Check sheet for the modelled part. Datum: model origin and axes. Units: mm. Face numbers are marked on the shaded views. A direction names the side the tool comes from. Round coordinates to 2 decimals unless told otherwise and drop trailing zeros. Write each loop counter-clockwise with the first axis right and the second up, starting at its lowest first coordinate (ties: lowest second). Pieces come first, ordered by that corner, then holes. Notation, with made-up numbers: (57, 62) -> (93, 62) arc R17 ccw to (93, 90) -> close; hole circle Ø5 at (-30, 31). An arc over 180 degrees is marked (long way). One line per item, written item: value.
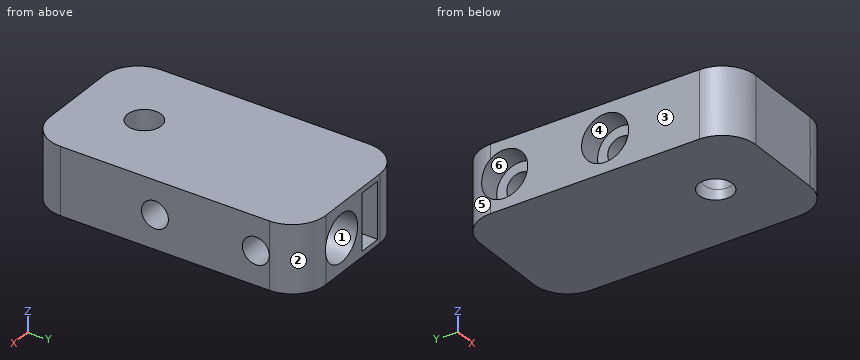
from build123d import *

# Parameters (mm, degrees)
CROQUIS1_W              = 10
CROQUIS1_H              = 41
SALIENTE_EXTRUIR1_DEPTH = 21.8
CROQUIS6_R              = 2
CORTAR_EXTRUIR2_DEPTH   = 21.8
CORTAR_EXTRUIR4_REACH   = 49.5
CROQUIS11_R             = 3.5
CROQUIS11_W             = 3.4
CROQUIS11_H             = 8.4
CORTAR_EXTRUIR5_REACH   = 49.5
CROQUIS12_R             = 2.5
REDONDEO1_R             = 5
CROQUIS13_R             = 3.5
CORTAR_EXTRUIR6_DEPTH   = 3.5
CROQUIS15_W             = 3.4
CROQUIS15_H             = 8.4
SALIENTE_EXTRUIR2_DEPTH = 13
CORTAR_EXTRUIR7_START   = -10
CROQUIS16_R             = 2.5
CORTAR_EXTRUIR7_DEPTH   = 10


with BuildPart() as part:
    # Croquis1 → Saliente-Extruir1 (new body)
    with BuildSketch(Plane(origin=(0, 0, 0), x_dir=(0, 0, -1), z_dir=(1, 0, 0))):
        with Locations((-5, -20.5)):
            Rectangle(CROQUIS1_W, CROQUIS1_H)
    extrude(amount=SALIENTE_EXTRUIR1_DEPTH)

    # Croquis6 → Cortar-Extruir2 (cut)
    with BuildSketch(Plane.ZY):
        with Locations((5, -22)):
            Circle(CROQUIS6_R)
        with Locations((5, -7)):
            Circle(CROQUIS6_R)
    extrude(amount=-CORTAR_EXTRUIR2_DEPTH, mode=Mode.SUBTRACT)

    # Croquis11 → Cortar-Extruir4 (cut, up to next)
    with BuildSketch(Plane.XZ.offset(41), mode=Mode.PRIVATE) as cortar_extruir4_sk1:
        with Locations(Location((13.4, 5, 0), (0, 0, 270))):
            Circle(CROQUIS11_R)
    cortar_extruir4_tool1 = extrude(cortar_extruir4_sk1.sketch, amount=-CORTAR_EXTRUIR4_REACH, mode=Mode.PRIVATE) & part.part
    # Croquis11 → Cortar-Extruir4 (cut, up to next)
    with BuildSketch(Plane.XZ.offset(41), mode=Mode.PRIVATE) as cortar_extruir4_sk2:
        with Locations((7.2, 5)):
            Rectangle(CROQUIS11_W, CROQUIS11_H)
    cortar_extruir4_tool2 = extrude(cortar_extruir4_sk2.sketch, amount=-CORTAR_EXTRUIR4_REACH, mode=Mode.PRIVATE) & part.part
    add(cortar_extruir4_tool1.solids().sort_by_distance((13.4, -41, 5))[0], mode=Mode.SUBTRACT)
    add(cortar_extruir4_tool2.solids().sort_by_distance((7.2, -41, 5))[0], mode=Mode.SUBTRACT)

    # Cortar-Extruir5: up to this face of the body (flat: up to its plane)
    cortar_extruir5_end = Plane(part.part.faces().sort_by_distance((10.9, -20.5, 10))[0])
    # Croquis12 → Cortar-Extruir5 (cut, up to the picked face)
    with BuildSketch(Plane(origin=(0, 0, 0), x_dir=(-1, 0, 0), z_dir=(0, 0, -1)), mode=Mode.PRIVATE) as cortar_extruir5_sk1:
        with Locations(Location((-10.9, -31, 0), (0, 0, 90))):
            Circle(CROQUIS12_R)
    cortar_extruir5_tool1 = split(extrude(cortar_extruir5_sk1.sketch, amount=-CORTAR_EXTRUIR5_REACH, mode=Mode.PRIVATE), bisect_by=cortar_extruir5_end, keep=Keep.BOTH, mode=Mode.PRIVATE)
    add(cortar_extruir5_tool1.solids().sort_by(Axis((10.9, -31, 0), (0, 0, 1)))[0], mode=Mode.SUBTRACT)

    # Redondeo1
    # the kernel refuses this fillet: 5 mm, written as the material it takes off along each edge
    with BuildSketch(Plane(origin=(21.8, -41, 22.5), x_dir=(0, 1, 0), z_dir=(0, 0, -1)), Plane(origin=(0, 0, -12.5), x_dir=(1, 0, 0), z_dir=(0, 0, 1))) as redondeo1_piece_1:
        with BuildLine():
            CenterArc((REDONDEO1_R, -REDONDEO1_R), REDONDEO1_R, 90, 90)
            Line((0, -REDONDEO1_R), (0, 0))
            Line((0, 0), (REDONDEO1_R, 0))
        make_face()
    extrude(amount=35, mode=Mode.SUBTRACT)
    with BuildSketch(Plane(origin=(21.8, 0, -12.5), x_dir=(-1, 0, 0), z_dir=(0, 0, 1)), Plane(origin=(0, -41, 22.5), x_dir=(0, 1, 0), z_dir=(0, 0, -1))) as redondeo1_piece_2:
        with BuildLine():
            CenterArc((REDONDEO1_R, REDONDEO1_R), REDONDEO1_R, 180, 90)
            Line((0, REDONDEO1_R), (0, 0))
            Line((0, 0), (REDONDEO1_R, 0))
        make_face()
    extrude(amount=35, mode=Mode.SUBTRACT)

    # Croquis13 → Cortar-Extruir6 (cut)
    with BuildSketch(Plane.ZY):
        with Locations((5, -7)):
            Circle(CROQUIS13_R)
        with Locations((5, -22)):
            Circle(CROQUIS13_R)
    extrude(amount=-CORTAR_EXTRUIR6_DEPTH, mode=Mode.SUBTRACT)

    # Croquis15 → Saliente-Extruir2 (add)
    with BuildSketch(Plane.XZ.offset(41)):
        with Locations((7.2, 5)):
            Rectangle(CROQUIS15_W, CROQUIS15_H)
        with BuildLine():
            ThreePointArc((16.8, 4.169337614), (16.9, 5), (16.8, 5.830662386))
            ThreePointArc((16.8, 5.830662386), (9.9, 5), (16.8, 4.169337614))
        make_face()
    extrude(amount=-SALIENTE_EXTRUIR2_DEPTH)

    # Croquis16 → Cortar-Extruir7 (cut)
    with BuildSketch(Plane.XY.offset(10).offset(CORTAR_EXTRUIR7_START)):
        with Locations(Location((10.9, -31, 0), (0, 0, 90))):
            Circle(CROQUIS16_R)
    extrude(amount=CORTAR_EXTRUIR7_DEPTH, mode=Mode.SUBTRACT)


solid = part.part
Item 1: Depth check by flat-ended pin: P1, Ø1, axis at x = 3, y = -24, coming from the -Z side; P2, Ø2, axis at y = -8, z = 5.5, coming from the -X side; P3, Ø1.7, axis at x = 7, z = 6, coming from the +Y side. Enter the tip coordinate at first touch or a pass-through.
Answer:
P1: stops at z = 0
P2: stops at x = 3.5
P3: stops at y = -28
Item 2: Tool access check on the marked faces 5 and 6. Record the directions out of +Z, -Z, +X, -X, +Y, -Y that give a thin tool (end or side, any length) a straight path to the whole face; none if there is none.
Answer:
face 5: +Z, -Z, -X, +Y
face 6: -X
Item 3: Sectioned sample at C-C on y = -13. Enter the section's corners in (x, z).
Answer:
outline: (0, 0) -> (21.8, 0) -> (21.8, 10) -> (0, 10) -> close; hole (5.5, 0.8) -> (8.9, 0.8) -> (8.9, 9.2) -> (5.5, 9.2) -> close; hole circle Ø7 at (13.4, 5)
Item 4: Sectioned sample at D-D on x = 17.5. Enter the section's corners in (y, z).
Answer:
outline: (-40.95, 0) -> (-0.05, 0) -> (-0.05, 10) -> (-40.95, 10) -> close; hole circle Ø4 at (-22, 5); hole circle Ø4 at (-7, 5)
Item 5: Sectioned sample at B-B on x = 9.5. Enter the section's corners in (y, z).
Answer:
outline: (-41, 0) -> (-33.07, 0) -> (-33.07, 10) -> (-41, 10) -> close; (-28.93, 0) -> (0, 0) -> (0, 10) -> (-28.93, 10) -> close; hole circle Ø4 at (-22, 5); hole circle Ø4 at (-7, 5)
Item 6: Mould release check, pull along X, two halves, no side actions. Record for the marked faces 1, 2, 3 and 4: pulls with the +X half, pulls with the -X half, needs draft (parallel to the pull), parting line crosses it, or undercut.
Answer:
face 1: undercut
face 2: pulls with the +X half
face 3: pulls with the -X half
face 4: needs draft
Item 7: Sectioned sample at A-A on y = -7. Enter the section's corners in (x, z), and give its area (3 significant figures).
Answer:
outline: (0, 0) -> (21.8, 0) -> (21.8, 3) -> (16.27, 3) arc R3.5 cw to (10.53, 3) -> (8.9, 3) -> (8.9, 0.8) -> (5.5, 0.8) -> (5.5, 3) -> (3.5, 3) -> (3.5, 1.5) -> (0, 1.5) -> close; (0, 8.5) -> (3.5, 8.5) -> (3.5, 7) -> (5.5, 7) -> (5.5, 9.2) -> (8.9, 9.2) -> (8.9, 7) -> (10.53, 7) arc R3.5 cw to (16.27, 7) -> (21.8, 7) -> (21.8, 10) -> (0, 10) -> close
area: 93.2 mm^2
Item 8: Thickness scan on line 1 (X direction, y = -16.5, z = 5); line 2 (X direction, y = -19.5, z = 5); line 3 (X direction, y = -31, z = 3.25). Record the ranges inside material, lowest first.
Answer:
line 1: x = 0 to 5.5, 8.9 to 9.9, 16.9 to 21.8
line 2: x = 3.5 to 5.5, 8.9 to 9.9, 16.9 to 21.8
line 3: x = 0 to 8.4, 13.4 to 21.8
